from build123d import *

# Parameters (mm, degrees)
F1_DEPTH = 12.7
F3_DEPTH = 7.62
F4_W     = 12.783553
F4_H     = 21.205658
F5_DEPTH = 5.08


with BuildPart() as f1:
    # F0 (on Top) → F1 (new body)
    with BuildSketch(Plane.XY):
        with BuildLine():
            Line((17.596183, -18.197764), (17.596183, 0))
            Line((17.596183, 0), (-17.596183, 0))
            Line((-17.596183, 0), (-17.596183, -18.197764))
            ThreePointArc((-17.596183, -18.197764), (0, -25.313717), (17.596183, -18.197764))
        make_face()
    extrude(amount=F1_DEPTH)

    # F2 (on Front) → F3 (join)
    with BuildSketch(Plane.XZ):
        with BuildLine():
            Line((-17.596183, 12.7), (17.596183, 12.7))
            Line((17.596183, 12.7), (17.596183, 68.321375))
            Line((17.596183, 68.321375), (5.865396, 68.321375))
            Line((5.865396, 68.321375), (5.865396, 41.663684))
            ThreePointArc((5.865396, 41.663684), (0, 35.798287), (-5.865396, 41.663684))
            Line((-5.865396, 41.663684), (-5.865396, 68.321375))
            Line((-5.865396, 68.321375), (-17.596183, 68.321375))
            Line((-17.596183, 68.321375), (-17.596183, 12.7))
        make_face()
    extrude(amount=F3_DEPTH)

    # F4 (on face) → F5 (cut)
    with BuildSketch(Plane.YZ.offset(17.596183)):
        with Locations((-6.391776, 10.602829)):
            Rectangle(F4_W, F4_H)
    extrude(amount=-F5_DEPTH, mode=Mode.SUBTRACT)


solid = f1.part
Input: part model. Units: mm. Frame: model coordinates. A direction names the side the tool comes from. Give positions to 0.01 mm unless a question says otherwise; leave off trailing zeros. Order: outer loops, then holes, each group sorted by start corner. A loop starts at its lowest first (then second) coordinate and runs counter-clockwise, first axis right, second up. Notation, with made-up numbers: M -20,-30 L 17,-30 A20 ccw 17,-17 Z; hole C 40,-9 d2. An arc over 180 degrees is marked long. Answer as a JSON object with one key per item and string values.
1. Cut plane A-A, the plane z = 62.5. Output: boundary loops of the cut face in (x, y), and give its area (3 significant figures).
Result sheet:
{"outline": "M -17.6,-7.62 L -5.87,-7.62 L -5.87,0 L -17.6,0 Z; M 5.87,-7.62 L 17.6,-7.62 L 17.6,0 L 5.87,0 Z", "area": "179 mm²"}
2. Reachability of faces 4 (the flat face through (12.516, -5, 8)), 5 (the flat face through (15, -4, 21.206)), 6 (the flat face through (5.865, -4, 55)) from +Z, -Z, +X, -X, +Y, -Y: full face, straight path, thin tool, end or side. Return the list, or none.
Result sheet:
{"face 4": "-Z, +X, +Y", "face 5": "-Z, +X, +Y, -Y", "face 6": "+Z, +Y, -Y"}
3. Cut plane C-C, the plane x = 0. Output: boundary loops of the cut face in (y, z), and give its area (3 significant figures).
Result sheet:
{"outline": "M -25.31,0 L 0,0 L 0,35.8 L -7.62,35.8 L -7.62,12.7 L -25.31,12.7 Z", "area": "497 mm²"}
4. Cut plane D-D, the plane z = 35. Output: boundary loops of the cut face in (x, y), and give its area (3 significant figures).
Result sheet:
{"outline": "M -17.6,-7.62 L 17.6,-7.62 L 17.6,0 L -17.6,0 Z", "area": "268 mm²"}
5. Ray query, line 1 (X direction, y = -5.75, z = 57.5); line 2 (Z direction, x = -11.5, y = -15); line 3 (Y direction, x = 6.5, z = 13.5). Return the intervals inside material, ascending. Write a range as [from, to].
Result sheet:
{"line 1": "[-17.6, -5.87], [5.87, 17.6]", "line 2": "[0, 12.7]", "line 3": "[-7.62, 0]"}
6. Pull-direction query (X, two-part tool) for faces 1 (the flat face through (-17.596, -5, 27)), 2 (the flat face through (-5.865, -4, 55)), 3 (the flat face through (17.596, -15, 6)); classes: +X half, -X half, draft (parallel to the pull), parting line (faces both ways), or undercut.
Result sheet:
{"face 1": "-X half", "face 2": "undercut", "face 3": "+X half"}
7. Cut plane B-B, the plane y = -3.25. Output: boundary loops of the cut face in (x, z), and give its area (3 significant figures).
Result sheet:
{"outline": "M -17.6,0 L 12.52,0 L 12.52,21.21 L 17.6,21.21 L 17.6,68.32 L 5.87,68.32 L 5.87,41.66 A5.87 cw -5.87,41.66 L -5.87,68.32 L -17.6,68.32 Z", "area": "1,930 mm²"}
8. First-contact query: P1, Ø2, axis at y = -9, z = 29, coming from the +X side; P2, Ø4, axis at x = 15.5, z = 5.5, coming from the +Y side; P3, Ø1.5, axis at x = 3, y = -18, coming from the -Z side; P4, Ø4, axis at x = -4.5, y = -18.5, coming from the +Z side. Flat tips, straight axial feed; report the tip coordinate or a pass-through.
Result sheet:
{"P1": "through", "P2": "y = -12.78", "P3": "z = 0", "P4": "z = 12.7"}
